Can you work these out from the model? Positions are in its coordinate system, mm. A direction names the side the tool comes from. Round coordinates to 2 decimals unless told otherwise and drop trailing zeros. Loops run counter-clockwise (first coordinate to the right, second up) from the corner with the lowest first, then second, coordinate; pieces in that order, holes last. Notation, with made-up numbers: (-36, 54.5) -> (-32, 54.5) arc R23 cw to (-32, 78.5) -> close; hole circle Ø4 at (80, 53). An arc over 180 degrees is marked (long way). Use a Markdown table: item, result.
from build123d import *

# Parameters (mm, degrees)
F0_W     = 70
F0_H     = 70
F0_R     = 3.5
F0_R_2   = 12.7
F1_DEPTH = 5
F2_W     = 50
F2_H     = 50
F2_W_2   = 35
F2_H_2   = 35
F3_DEPTH = 35
F4_R     = 13.4
F4_R_2   = 12.7
F5_DEPTH = 2.5


# Not quite as in the source:
# - a feature names something its author has since deleted; it is built from what else it names


with BuildPart() as f1:
    # F0 (on Top) → F1 (new body)
    with BuildSketch(Plane.XY):
        Rectangle(F0_W, F0_H)
        with Locations((28.5, -28.5)):
            Circle(F0_R, mode=Mode.SUBTRACT)
        with Locations((-28.5, 28.5)):
            Circle(F0_R, mode=Mode.SUBTRACT)
        Circle(F0_R_2, mode=Mode.SUBTRACT)
    extrude(amount=F1_DEPTH)

    # F2 (on face) → F3 (join)
    with BuildSketch(Plane.XY.offset(5)):
        Rectangle(F2_W, F2_H)
        Rectangle(F2_W_2, F2_H_2, mode=Mode.SUBTRACT)
    extrude(amount=F3_DEPTH)

    # F4 (on face) → F5 (cut)
    with BuildSketch(Plane(origin=(0, 0, 0), x_dir=(1, 0, 0), z_dir=(0, 0, -1))):
        Circle(F4_R)
        Circle(F4_R_2, mode=Mode.SUBTRACT)
    extrude(amount=-F5_DEPTH, mode=Mode.SUBTRACT)


solid = f1.part
1. I want a section at A-A (y = 28.5). Please give me the cut outline in (x, z), plus the area to 3 significant figures.
Answer sheet:
| item | result |
|---|---|
| outline | (-35, 0) -> (-32, 0) -> (-32, 5) -> (-35, 5) -> close; (-25, 0) -> (35, 0) -> (35, 5) -> (-25, 5) -> close |
| area | 315 mm² |
2. I need wall thicknesses on line 1 (X direction, y = 0, z = 1.9); line 2 (X direction, y = -10.5, z = 30); line 3 (Y direction, x = 0, z = 3). Which ranges of each line are inside material? Lowest first, please.
Answer sheet:
| item | result |
|---|---|
| line 1 | x = -35 to -13.4, 13.4 to 35 |
| line 2 | x = -25 to -17.5, 17.5 to 25 |
| line 3 | y = -35 to -12.7, 12.7 to 35 |
3. I want a section at D-D (x = -24). Please give me the cut outline in (y, z).
Answer sheet:
| item | result |
|---|---|
| outline | (-35, 0) -> (35, 0) -> (35, 5) -> (25, 5) -> (25, 40) -> (-25, 40) -> (-25, 5) -> (-35, 5) -> close |
4. I want a section at B-B (x = 0). Please give me the cut outline in (y, z), plus the area to 4 significant figures.
Answer sheet:
| item | result |
|---|---|
| outline | (-35, 0) -> (-13.4, 0) -> (-13.4, 2.5) -> (-12.7, 2.5) -> (-12.7, 5) -> (-17.5, 5) -> (-17.5, 40) -> (-25, 40) -> (-25, 5) -> (-35, 5) -> close; (12.7, 2.5) -> (13.4, 2.5) -> (13.4, 0) -> (35, 0) -> (35, 5) -> (25, 5) -> (25, 40) -> (17.5, 40) -> (17.5, 5) -> (12.7, 5) -> close |
| area | 744.5 mm² |
5. Which directions (+Z, -Z, +X, -X, +Y, -Y) give clear straight access to the entire face, cutting with the end or side of a thin tool? Please do faces 5 (the flat face through (17.5, 0, 22)), 6 (the flat face through (25, 0, 22)), 7 (the cylindrical face through (-13.387, -0.589, 1.232)).
Answer sheet:
| item | result |
|---|---|
| face 5 | +Z |
| face 6 | +Z, +X, +Y, -Y |
| face 7 | -Z |
6. Will these pins go through, and if not, where does the flat tip stop? pin 1 Ø10 at (x, z) = (3, 17) entering from +Y; pin 2 Ø5 at (x, z) = (-7.5, 29) entering from -Y; pin 3 Ø5.5 at (x, y) = (-28.5, 28.5) entering from +Z; pin 4 Ø4 at (y, z) = (-14.5, 30.5) entering from -X.
Answer sheet:
| item | result |
|---|---|
| pin 1 | stops at y = 25 |
| pin 2 | stops at y = -25 |
| pin 3 | passes through |
| pin 4 | stops at x = -25 |
7. If we mould it in two halves opening along Y, with no side actions, what happens to faces 1 (the cylindrical face through (-2.75, -12.4, 3.73)), 2 (the flat face through (0, -25, 22)), 3 (the flat face through (-35, 0, 2)), 4 (the flat face through (0, -17.5, 22))? For each: +Y half, -Y half, draft (parallel to the pull), parting line (faces both ways), or undercut.
Answer sheet:
| item | result |
|---|---|
| face 1 | undercut |
| face 2 | -Y half |
| face 3 | draft |
| face 4 | undercut |
8. I want a section at C-C (z = 12.5). Please give me the cut outline in (x, y), plus the area to 4 significant figures.
Answer sheet:
| item | result |
|---|---|
| outline | (-25, -25) -> (25, -25) -> (25, 25) -> (-25, 25) -> close; hole (-17.5, -17.5) -> (17.5, -17.5) -> (17.5, 17.5) -> (-17.5, 17.5) -> close |
| area | 1,275 mm² |
